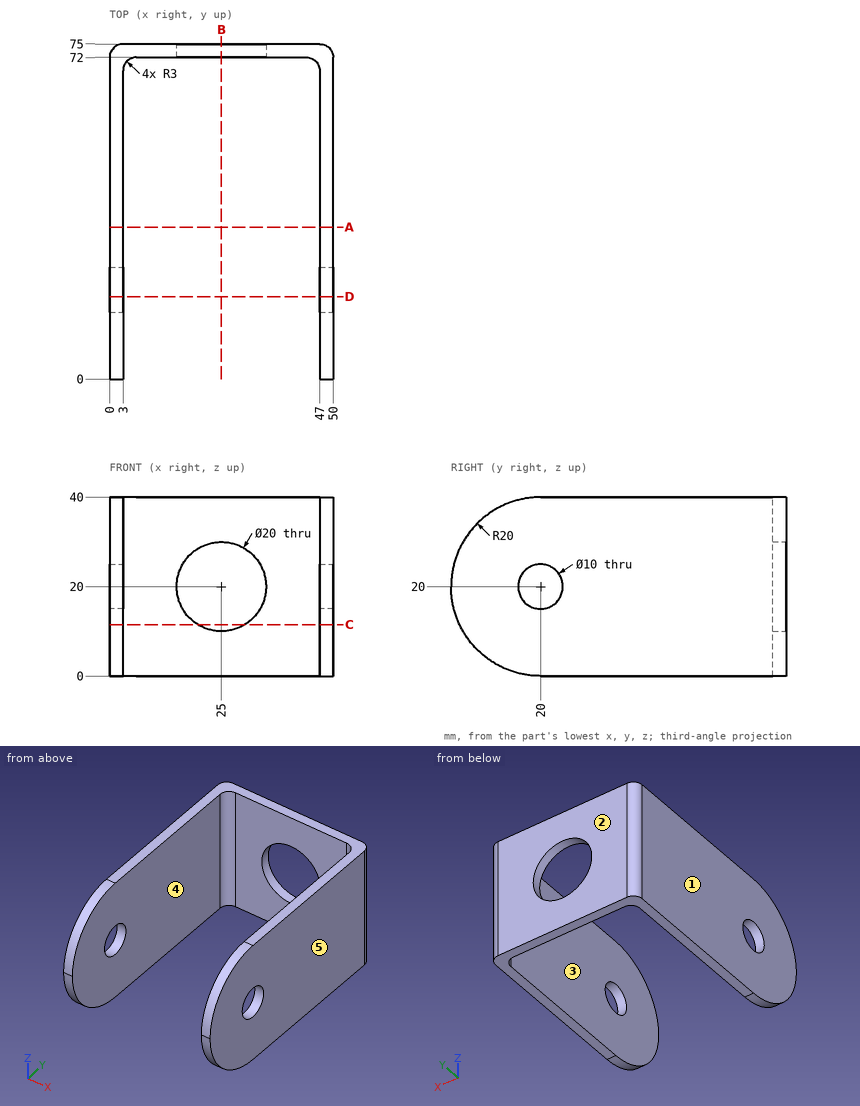
Study the drawing (mm; zero at the part's minimum x, y, z) and answer. A direction names the side the tool comes from. Coordinates: 2 decimals unless noted, no trailing zeros. Loops run counter-clockwise (first coordinate to the right, second up) from the corner with the lowest first, then second, coordinate; pieces in that order, holes last. Notation, with made-up numbers: M -37.5,11.25 L -9.5,11.25 A24 cw -9.5,41.25 Z; hole C 7.25,-40 d3. An arc over 180 degrees is marked long. Answer in a Markdown table with one row per item. Add a question column.
1. Find section B-B, the plane x = 25. Write down the section's boundary in (y, z).
2. Find section A-A, the plane y = 34. Write down the section's boundary in (x, z).
3. Find section D-D, the plane y = 18.5. Write down the section's boundary in (x, z), then the cut area to 3 significant figures.
4. Consider L1, parallel to X at y = 64.5, z = 33; L2, parallel to Z at x = 25, y = 73; L3, parallel to Y at x = 33, z = 10.5. Determine where each line is inside the solid, lowest interval first.
5. A flat-ended cylindrical pin translates along its axis: P1, Ø4, axis at x = 7, z = 16, coming from the -Y side. Find the tip coordinate at first contact, or state that the pin passes through.
6. Find section C-C, the plane z = 11.5. Write down the section's boundary in (x, y), then the cut area to 3 significant figures.
7. The mould has two halves that part along X. Classify the marked faces 1, 2 and 3: pulls with the +X half, pulls with the -X half, needs draft (parallel to the pull), parting line crosses it, or undercut.
8. A tool of negligible diameter and unlimited length cuts with its end or side. For the marked faces 4 and 5, from which of +Z, -Z, +X, -X, +Y, -Y can it reach the whole face along a straight path? Write none if from no direction.
Reported:
| question | item | result |
|---|---|---|
| 1 | outline | M 72,0 L 75,0 L 75,10 L 72,10 Z; M 72,30 L 75,30 L 75,40 L 72,40 Z |
| 2 | outline | M 0,0 L 3,0 L 3,40 L 0,40 Z; M 47,0 L 50,0 L 50,40 L 47,40 Z |
| 3 | outline | M 0,0.06 L 3,0.06 L 3,15.23 L 0,15.23 Z; M 0,24.77 L 3,24.77 L 3,39.94 L 0,39.94 Z; M 47,0.06 L 50,0.06 L 50,15.23 L 47,15.23 Z; M 47,24.77 L 50,24.77 L 50,39.94 L 47,39.94 Z |
| 3 | area | 182 mm^2 |
| 4 | L1 | x = 0 to 3, 47 to 50 |
| 4 | L2 | z = 0 to 10, 30 to 40 |
| 4 | L3 | y = 72 to 75 |
| 5 | P1 | stops at y = 71.83 |
| 6 | outline | M 0,1.9 L 3,1.9 L 3,69 A3 cw 6,72 L 19.73,72 L 19.73,75 L 3,75 A3 ccw 0,72 Z; M 30.27,72 L 44,72 A3 cw 47,69 L 47,1.9 L 50,1.9 L 50,72 A3 ccw 47,75 L 30.27,75 Z |
| 6 | area | 539 mm^2 |
| 7 | face 1 | pulls with the -X half |
| 7 | face 2 | needs draft |
| 7 | face 3 | undercut |
| 8 | face 4 | +Z, -Z, -Y |
| 8 | face 5 | +Z, -Z, +X, +Y, -Y |
